For this review, take the finished solid that the model builds, in its own axes (mm). A direction names the side the tool comes from. Coordinates: 2 decimals unless noted, no trailing zeros. Order: outer loops, then holes, each group sorted by start corner. A loop starts at its lowest first (then second) coordinate and runs counter-clockwise, first axis right, second up.
Autodesk Inventor part; units mm, degrees
ref_plane "Work Plane1" through (-20.2583, -25.7942, 0) normal (0, 0, 1) x (1, 0, 0)
ref_plane "Work Plane4" through (8.9999, -18.0001, 0) normal (1, 0, 0) x (0, 0, -1)
ref_plane "YZ Plane" through (0, 0, 0) normal (1, 0, 0) x (0, 1, 0)
sketch "Sketch1" plane through (0, 0, 0) normal (0, 0, 1) x (1, 0, 0)
  circle A0 centre (-0.0001, 55.0001) radius 2.5
  line L0 (-9, 60.0001) -> (-9, 34.0001)
  line L1 (-9, 34.0001) -> (-5.0001, 34.0001)
  line L2 (-5.0001, 34.0001) -> (-5.0001, 45.0001)
  line L3 (-5.0001, 45.0001) -> (4.9999, 45.0001)
  line L4 (4.9999, 45.0001) -> (4.9999, 34.0001)
  line L5 (4.9999, 34.0001) -> (8.9999, 34.0001)
  line L6 (8.9999, 34.0001) -> (8.9999, 60.0001)
  line L7 (8.9999, 60.0001) -> (-9, 60.0001)
  line L8 (-9, 8) -> (-9, -18)
  line L9 (-5, -18) -> (-5, -8)
  circle A1 centre (-0.0001, -13.0001) radius 2.5
  line L10 (8.9999, -18.0001) -> (8.9999, 7.9999)
  line L11 (8.9999, 7.9999) -> (4.9999, 7.9999)
  line L12 (4.9999, 7.9999) -> (4.9999, 2.5001)
  line L13 (5, -3) -> (-5.0001, -3.0001)
  line L14 (-5.0001, -3.0001) -> (-5.0001, 7.9999)
  line L15 (-5.0001, 7.9999) -> (-9, 7.9999)
  line L16 (-9, -18.0001) -> (8.9999, -18.0001)
  line L17 (8.9999, 60.0001) -> (-9, 60.0001)
  line L18 (-9, 60.0001) -> (-9, -18)
  line L19 (-9, -18) -> (8.9999, -18)
  line L20 (8.9999, -18) -> (8.9999, 60.0001)
  circle A2 centre (-0.0001, 55.0001) radius 2.5
  circle A3 centre (-0.0001, -13.0001) radius 2.5
  line L21 (-9, 7.9999) -> (-9, -18.0001)
  line L22 (4.9999, 2.5001) -> (5, -3)
  point P0 (0, 0)
  dimension "d0" = 4
  dimension "d1" = 0
extrude "Extrusion1" add sketch "Sketch1" along normal blind 4
sketch "Sketch2" plane through (0, 0, 4) normal (0, 0, 1) x (1, 0, 0)
  circle A0 centre (-55.3, -73.0192) radius 2.5
  circle A1 centre (-55.3001, 115.0193) radius 2.5
  line L0 (-55.3, -73.0192) -> (33.584, 75.4143)
  line L1 (-55.3001, 115.0193) -> (26.1085, -20.9304)
  line L2 (-9, 60) -> (-9, -18)
  line L3 (-9, 21) -> (62.9573, 21)
  line L4 (1, 21) -> (-7.5794, 15.8625)
  line L5 (-55.3001, 115.0193) -> (-50.1626, 106.4399)
  line L6 (-50.1626, 106.4399) -> (-41.5832, 111.5774)
  line L7 (-50.1626, 106.4399) -> (-58.742, 101.3024)
  line L8 (-7.5794, 15.8625) -> (-58.742, 101.3024)
  line L9 (1, 21) -> (9.5794, 26.1375)
  line L10 (9.5794, 26.1375) -> (-41.5832, 111.5774)
  line L11 (1, 21) -> (-7.5794, 26.1375)
  line L12 (1, 21) -> (9.5794, 15.8625)
  line L13 (-55.3, -73.0192) -> (-50.1625, -64.4398)
  line L14 (-93.1275, -68.5) -> (-47.8, -94.6699)
  line L15 (-50.1625, -64.4398) -> (-41.5831, -69.5773)
  line L16 (-50.1625, -64.4398) -> (-58.742, -59.3023)
  line L17 (-41.5831, -69.5773) -> (9.5794, 15.8625)
  line L18 (-7.5794, 26.1375) -> (-58.742, -59.3023)
  line L19 (-10.6558, 21) -> (6.503, 31.2749)
  line L20 (-10.6558, 21) -> (6.503, 10.7251)
  circle A2 centre (-0.0001, -13.0001) radius 2.5
  circle A3 centre (-0.0001, -13.0001) radius 5
  circle A4 centre (-0.0001, 55.0001) radius 2.5
  circle A5 centre (-0.0001, 55.0001) radius 5
  line L21 (8.9999, 60.0001) -> (-9, 60.0001)
  line L22 (-9, -18.0001) -> (8.9999, -18.0001)
  line L23 (-20.2607, 4.9602) -> (12.7451, -14.8042)
  line L24 (-20.2607, 37.0398) -> (12.7451, 56.8042)
  line L25 (-20.2607, 4.9602) -> (-22.8345, 6.5014)
  line L26 (-9, 21) -> (-33.1607, 21)
  line L27 (-22.8345, 6.5014) -> (-14.1525, 21)
  line L28 (-20.2607, 37.0398) -> (-22.8345, 35.4986)
  line L29 (-22.8345, 35.4986) -> (-14.1525, 21)
  line L30 (6.503, 10.7251) -> (8.9999, 9.2299)
  line L31 (8.9999, -18.0001) -> (8.9999, 60.0001)
  line L32 (6.503, 31.2749) -> (8.9999, 32.7701)
  line L33 (8.9999, 32.7701) -> (-0.605, 48.8099)
  line L34 (8.9999, 9.2299) -> (-0.605, -6.8099)
  line L35 (8.9999, 32.7701) -> (8.9999, 9.2299)
  line L36 (-22.8345, 6.5014) -> (-22.8345, 35.4986)
  point P0 (0, 0)
  point P1 (-20.2607, 37.0398)
  point P2 (6.503, 10.7251)
  point P3 (-3.1018, -5.3148)
  point P4 (8.524, 8.4352)
  point P5 (7.516, 10.1185)
  point P6 (-3.1019, 47.3148)
  point P7 (6.503, 31.2749)
  point P8 (-2.0764, 26.1375)
  point P9 (-11.6813, 42.1773)
  point P10 (6.8279, 11.2676)
  point P11 (8.9999, 14.8947)
  point P12 (8.9999, 16.2096)
  point P13 (6.503, 10.7251)
  point P14 (8.9999, 25.7904)
  point P15 (6.503, 31.2749)
  point P16 (8.9999, 27.1053)
  point P17 (8.9999, 32.7701)
  point P18 (8.9999, 32.7704)
  point P19 (8.9999, 9.2299)
  point P20 (8.9999, 7.6404)
  point P21 (8.9999, 9.2296)
  point P22 (8.9999, 54.5615)
  point P23 (8.9999, -12.5615)
  dimension "d0" = 4
  dimension "d1" = 0
  dimension "d2" = 10
  dimension "d3" = 10
  dimension "d4" = 10
  dimension "d5" = 10
  dimension "d6" = 10
  dimension "d7" = 10
  dimension "d8" = 10
  dimension "d9" = 10
  dimension "d10" = 10
  dimension "d11" = 10
  dimension "d12" = 10
  dimension "d13" = 20
  dimension "d14" = 20
  dimension "d15" = 3
  dimension "d16" = 3
extrude "Extrusion2" add sketch "Sketch2" along normal blind 20 contours L25 L27 L26 L18 | L20 L4 L0 | L0 L1 L17 L20 | L26 L29 L28 L8 | L26 L2 L20 | L19 L2 L26 | L17 L30 L1 L34 L23 | L1 L19 L10 L0 | L11 L19 L1 | L12 L31 L17 L1 | L4 L20 L2 L3 | L9 L31 L3 | L0 L10 L31 L9 | L3 L2 L19 L11 | L3 L31 L12 | L17 L1 L30 | L34 L1 L31 L23 | L10 L32 L0 | L0 L32 L31 L10 | L17 L31 L30 L1 | L30 L34 L1 | L34 L31 L1 | L32 L10 L24 L33 L0 | L0 L33 L32 | L33 L24 L31 L0 | L0 L31 L33
sketch "Sketch3" plane through (0, 0, 4) normal (0, 0, -1) x (-1, 0, 0)
  line L0 (10.6558, 21) -> (20.2607, 37.0398)
  line L1 (20.2607, 37.0398) -> (8.9915, 37.0398)
  line L2 (20.2607, 4.9602) -> (10.6558, 21)
  line L3 (20.2607, 4.9602) -> (9, 4.9602)
  line L4 (9, 20.0085) -> (9, -18)
  line L5 (22.8345, 35.4986) -> (14.1525, 21)
  line L6 (22.8345, 6.5014) -> (20.2607, 4.9602)
  line L7 (22.8345, 35.4986) -> (22.8345, 6.5014)
  line L8 (9, 60) -> (9, -18)
  line L9 (10.6558, 21) -> (9, 20.0085)
  line L10 (9, 21.9915) -> (10.6558, 21)
  line L11 (22.8345, 6.5014) -> (20.2607, 4.9602)
  line L12 (14.1525, 21) -> (22.8345, 6.5014)
  line L13 (22.8345, 35.4986) -> (14.1525, 21)
  line L14 (20.2607, 37.0398) -> (22.8345, 35.4986)
  line L15 (10.6558, 21) -> (20.2607, 37.0398)
  line L16 (20.2607, 4.9602) -> (10.6558, 21)
  line L17 (-8.9999, 60.0001) -> (9, 60.0001)
  line L18 (-8.9999, -18.0001) -> (-8.9999, 60.0001)
  line L19 (9, -18.0001) -> (-8.9999, -18.0001)
  circle A0 centre (0.0001, -13.0001) radius 2.5
  circle A1 centre (0.0001, 55.0001) radius 2.5
  line L20 (9, 60.0001) -> (9, -18.0001)
  point P0 (0, 0)
  point P1 (9, 37.0398)
  dimension "d0" = 4
  dimension "d1" = 0
ref_plane "Work Plane1" through (-20.2583, -25.7942, 0) normal (0, 0, 1) x (1, 0, 0)
extrude "Extrusion3" add sketch "Sketch3" along normal up to surface (4 mm away) contours L10 L8 L1 L0 | L0 L14 L5 L12 L6 L2 | L2 L3 L4 L9 | L9 L8 L10 | L7 L12 L5
ref_plane "Work Plane4" through (8.9999, -18.0001, 0) normal (1, 0, 0) x (0, 0, -1)
sketch "Sketch12" plane through (0, 0, 24) normal (0, 0, 1) x (1, 0, 0)
  line L0 (-3.1018, -5.3148) -> (8.9999, -12.5615)
  line L1 (-14.1525, 21) -> (-22.8345, 6.5014)
  line L2 (8.9999, -12.5615) -> (-22.8345, 6.5014)
  line L3 (-22.8345, 6.5014) -> (-14.1525, 21)
  line L4 (-22.8345, 35.4986) -> (-14.1525, 21)
  line L5 (-14.1525, 21) -> (-22.8345, 35.4986)
  line L6 (-22.8345, 35.4986) -> (8.9999, 54.5615)
  line L7 (8.9999, 54.5615) -> (8.9999, -12.5615)
  point P0 (0, 0)
extrude "Extrusion12" add sketch "Sketch12" along normal blind 3
sketch "Sketch13" plane through (0, 0, 27) normal (0, 0, 1) x (1, 0, 0)
  line L0 (8.9999, -12.5615) -> (8.9999, 54.5615)
  line L1 (8.9999, 21) -> (14.9999, 21)
  line L2 (8.9999, 21) -> (8.9999, 6)
  line L3 (8.9999, 21) -> (8.9999, 36)
  arc A0 (8.9999, 6) -> (8.9999, 36) centre (-6.7501, 21) ccw
  point P0 (0, 0)
  dimension "d52" = 6
  dimension "d53" = 15
  dimension "d54" = 15
extrude "Extrusion13" add sketch "Sketch13" against normal up to surface (27 mm away)
sketch "Sketch14" plane through (0, 0, 27) normal (0, 0, 1) x (1, 0, 0)
  arc A0 (8.9999, 6) -> (8.9999, 36) centre (-6.7501, 21) ccw
  line L0 (14.9999, 21) -> (7.9999, 21)
  circle A1 centre (7.9999, 21) radius 2.5
  point P0 (0, 0)
  dimension "d57" = 7
  dimension "d58" = 5
extrude "Extrusion14" cut sketch "Sketch14" against normal up to surface (23 mm away)
sketch "Sketch15" plane through (8.9999, -18.0001, 4) normal (1, 0, 0) x (0, 0, -1)
  line L0 (-23, 54.0001) -> (-23, 24.0001)
  line L1 (-23, 39.0001) -> (-10, 39.0001)
  line L2 (0, 39.0001) -> (-20, 39.0001)
  line L3 (-17.5, 31.5001) -> (-2.5, 31.5001)
  line L4 (-2.5, 31.5001) -> (-2.5, 46.5001)
  line L5 (-2.5, 46.5001) -> (-17.5, 46.5001)
  line L6 (-17.5, 46.5001) -> (-17.5, 31.5001)
  line L7 (-17.5, 31.5001) -> (-2.5, 46.5001) construction
  line L8 (-2.5, 31.5001) -> (-17.5, 46.5001) construction
  point P0 (4, 18.0001)
  dimension "d61" = 15
  dimension "d62" = 15
extrude "Extrusion15" cut sketch "Sketch15" along normal blind 10 and the other way blind 7
sketch "Sketch16" plane through (0, 0, 27) normal (0, 0, 1) x (1, 0, 0)
  line L0 (-3.1018, -5.3148) -> (6.503, 10.7251)
  line L1 (6.503, 31.2749) -> (-3.1019, 47.3148)
  line L2 (-3.1018, -5.3148) -> (-1.386, -6.3423)
  line L3 (-22.8345, 6.5014) -> (8.9999, -12.5615)
  line L4 (-1.386, -6.3423) -> (4.4507, 3.4048)
  line L5 (8.9999, -12.5615) -> (8.9999, 6)
  line L6 (8.9999, 6) -> (-9.8503, 6)
  line L7 (4.4507, 3.4048) -> (6.0048, 6)
  line L8 (-22.8345, 35.4986) -> (-14.1525, 21)
  line L9 (-14.1525, 21) -> (17.1457, 21)
  line L10 (-22.8345, 35.4986) -> (8.9999, 54.5615)
  line L11 (-1.386, 48.3423) -> (4.4507, 38.5952)
  line L12 (8.9999, 54.5615) -> (8.9999, 36)
  line L13 (8.9999, 36) -> (-9.8503, 36)
  line L14 (4.4507, 38.5952) -> (6.0048, 36)
  point P0 (0, 0)
  dimension "d67" = 2
extrude "Extrusion16" cut sketch "Sketch16" against normal up to surface (23 mm away) contours L4 L7 L6 L5 L3 | L14 L11 L10 L12 L13
sketch "Sketch17" plane through (6.0048, 6, 27) normal (0.8579416, -0.5137472, 0) x (0, 0, -1)
  line L0 (0, 2.5134) -> (0, -14.3859)
  line L1 (0, -8.2326) -> (13, -8.2326)
  circle A0 centre (13, -8.2326) radius 1.5
  point P0 (27, -8.2326)
  dimension "d71" = 13
  dimension "d72" = 3
extrude "Extrusion17" cut sketch "Sketch17" against normal through all
sketch "Sketch18" plane through (6.0048, 36, 27) normal (0.8579416, 0.5137472, 0) x (0, 0, -1)
  line L0 (23, 14.3859) -> (0, 14.3859)
  line L1 (0, 14.3859) -> (0, 8.2329)
  line L2 (0, 14.3859) -> (0, -2.5134)
  line L3 (0, 8.2329) -> (13, 8.2329)
  circle A0 centre (13, 8.2329) radius 1.5
  point P0 (27, -27.801)
  dimension "d75" = 6.153
  dimension "d76" = 13
  dimension "d77" = 3
extrude "Extrusion18" cut sketch "Sketch18" against normal through all
fillet "Fillet1" radius 2 4 edges at (2.3094, 42.1711, 27) (2.3094, -0.1711, 27) (-18.4935, 13.7507, 27) (-18.4935, 28.2493, 27)
properties part number "2020_top_guide_mnt" material "PET Plastic"
1. Machinability: for faces 4 (the face through (8, 21, 4)), 5 (the face through (10, 23, 21.5)), 6 (the face through (-7, 34, 24)), which of the approach directions +Z, -Z, +X, -X, +Y, -Y give a long, thin tool a straight path to every point of the face, cutting with its end or side? Answer none if there is none.
Answer below:
face 4: +Z
face 5: +X
face 6: none
2. Clearance check with flat-ended pins moving along their axes: pin 1 Ø3 at (x, z) = (6.5, 15.5) entering from -Y; pin 2 Ø6.5 at (x, y) = (8, 21) entering from +Z; pin 3 Ø4.5 at (y, z) = (24, 15.5) entering from +X; pin 4 Ø6 at (x, z) = (5.5, 16) entering from +Y. State where each tip first meets the part, or that it passes through.
Answer below:
pin 1: stops at y = 4.32
pin 2: stops at z = 27
pin 3: stops at x = 2
pin 4: stops at y = 41.85
3. To check wall thickness, follow L1, parallel to Y at x = 9, z = 14.25; L2, parallel to Z at x = 13, y = 24.5; L3, parallel to Z at x = -7, y = 32. State the ranges of each line that lie inside material, in increasing order.
Answer below:
L1: y = 6 to 13.5, 28.5 to 36
L2: z = 0 to 6.5, 21.5 to 27
L3: z = 0 to 4, 24 to 27
4. Take a section at C-C, the plane x = -7. Give the boundary of the cut face in (y, z), plus the area to 3 significant figures.
Answer below:
outline: (-18, 0) - (60, 0) - (60, 4) - (23.19, 4) - (23.19, 24) - (44.98, 24) - (44.98, 27) - (-2.98, 27) - (-2.98, 24) - (18.81, 24) - (18.81, 4) - (-18, 4) - close
area: 543 mm2
5. The part is to be moulded in two halves that separate along Y. For faces 1 (the face through (-3, 21, 27)), 2 (the face through (-17.73, 13.85, 26.43)), 3 (the face through (8, 6, 16)), say which applies: +Y half, -Y half, draft (parallel to the pull), parting line (faces both ways), or undercut.
Answer below:
face 1: draft
face 2: undercut
face 3: -Y half
